Source: CAD feature listing. Evaluate the final solid. Frame: model axes, mm. A direction names the side the tool comes from. Round coordinates to 2 decimals unless told otherwise and drop trailing zeros. Order: outer loops, then holes, each group sorted by start corner. A loop starts at its lowest first (then second) coordinate and runs counter-clockwise, first axis right, second up. Notation, with made-up numbers: (71.5, -19.5) - (90.5, -19.5) arc R21 cw to (90.5, -12.5) - close; hole circle Ø8 at (12, 83.5). An arc over 180 degrees is marked (long way). Return JSON: item names as keys, results as strings. Group by question number.
1) Section D-D, the plane z = -45. Return loops of the section in (x, y).
2) Ray query, line 1 (Y direction, x = 0, z = 257); line 2 (X direction, y = -2, z = 112); line 3 (Z direction, x = -43, y = -11). Return the intervals inside material, ascending. Write a range as from..to.
3) Contact query for flat-ended pins moving along their axis: P1, Ø4, axis at x = 17, z = 372.5, coming from the +Y side; P2, Ø2, axis at y = 11, z = 375, coming from the -X side; P3, Ø8, axis at x = -6, y = -19, coming from the -Z side. Output: stop coordinate, or through.
4) Section C-C, the plane z = 104. Return loops of the section in (x, y), plus the area to 3 significant figures.
5) Mould query, pull axis X, two halves, no side actions, for faces 4 (the flat face through (1, -10, -30)), 5 (the cylindrical face through (47.69, 15.02, 246.5)), 6 (the flat face through (0, 0, 30)). Classes: pulls with the +X half, pulls with the -X half, needs draft (parallel to the pull), parting line crosses it, or undercut.
6) Section B-B, the plane y = 0. Return loops of the section in (x, z), plus the area to 3 significant figures.
7) Section A-A, the plane x = 0. Return loops of the section in (y, z).
8) Access query for faces 1 (the flat face through (1, 10, -30)), 2 (the cylindrical face through (-4.336, -19.524, 261.71)), 3 (the cylindrical face through (0, 0, -55)). Directions: +Z, -Z, +X, -X, +Y, -Y. A direction counts if a zero-diameter tool reaches every point of the face in a straight line with its end or side. Return the directions, or none.
```python
from build123d import *

# Parameters (mm, degrees)
SKETCH1_R           = 50
BOSS_EXTRUDE1_DEPTH = 500
SKETCH2_R           = 10
BOSS_EXTRUDE2_DEPTH = 10
SHELL1_START        = 30
SHELL1_OUTLINE_R    = 20
SHELL1_DEPTH        = 470


# Read off the part's stored shape, not the designer's step: Shell1
with BuildPart() as part:
    # Sketch1 → Boss-Extrude1 (new body)
    with BuildSketch(Plane.XY):
        Circle(SKETCH1_R)
    extrude(amount=BOSS_EXTRUDE1_DEPTH)

    # Sketch2 → Boss-Extrude2 (add, symmetric)
    with BuildSketch(Plane(origin=(0, 0, 0), x_dir=(1, 0, 0), z_dir=(0, 1, 0))):
        with BuildLine():
            Line((-45, 0), (-28.708286934, 53.708286934))
            ThreePointArc((-28.708286934, 53.708286934), (0, 75), (28.708286934, 53.708286934))
            Line((28.708286934, 53.708286934), (45, 0))
            Line((45, 0), (-45, 0))
        make_face()
        with Locations(Location((0, 45, 0), (0, 0, 270))):
            Circle(SKETCH2_R, mode=Mode.SUBTRACT)
    extrude(amount=BOSS_EXTRUDE2_DEPTH, both=True)

    # Shell1 outline → Shell1 (cut)
    with BuildSketch(Plane.XY.offset(SHELL1_START)):
        Circle(SHELL1_OUTLINE_R)
    extrude(amount=SHELL1_DEPTH, mode=Mode.SUBTRACT)


solid = part.part
```
Geometry check:
{
 "1": {"outline": "(-31.35, -10) - (-10, -10) - (-10, 10) - (-31.35, 10) - close; (10, -10) - (31.35, -10) - (31.35, 10) - (10, 10) - close"},
 "2": {"line 1": "-50..-20, 20..50", "line 2": "-49.96..-19.9, 19.9..49.96", "line 3": "0..500"},
 "3": {"P1": "y = 47.7", "P2": "x = -48.99", "P3": "z = 0"},
 "4": {"outline": "circle Ø100 at (0, 0); hole circle Ø40 at (0, 0)", "area": "6,600 mm2"},
 "5": {"face 4": "needs draft", "face 5": "parting line crosses it", "face 6": "undercut"},
 "6": {"outline": "(-50, 0) - (-45, 0) - (-28.71, -53.71) arc R30 ccw to (28.71, -53.71) - (45, 0) - (50, 0) - (50, 500) - (20, 500) - (20, 30) - (-20, 30) - (-20, 500) - (-50, 500) - close; hole circle Ø20 at (0, -45)", "area": "35,700 mm2"},
 "7": {"outline": "(-50, 0) - (-10, 0) - (-10, -35) - (10, -35) - (10, 0) - (50, 0) - (50, 500) - (20, 500) - (20, 30) - (-20, 30) - (-20, 500) - (-50, 500) - close; (-10, -75) - (10, -75) - (10, -55) - (-10, -55) - close"},
 "8": {"face 1": "-Z, +X, -X, +Y", "face 2": "+Z", "face 3": "+Y, -Y"}
}
